```python
from build123d import *

# Parameters (mm, degrees)
F1_R     = 3.5625
F3_DEPTH = 12
F5_DEPTH = 3
F6_W     = 2.2875
F6_H     = 3.4472514316
F8_DEPTH = 2


with BuildPart() as f3:
    # F1 (on Top) → F3 (new body)
    with BuildSketch(Plane.XY):
        Circle(F1_R)
    extrude(amount=F3_DEPTH)

    # F2 (on Top) → F5 (join)
    with BuildSketch(Plane.XY):
        with BuildLine():
            ThreePointArc((-7.5208044782, -3), (-7.809575399, -2.1384648903), (-8, -1.25))
            ThreePointArc((-8, -1.25), (-9.25, 0), (-8, 1.25))
            ThreePointArc((-8, 1.25), (-7.809575399, 2.1384648903), (-7.5208044782, 3))
            Line((-7.5208044782, 3), (-9.25, 3))
            ThreePointArc((-9.25, 3), (-12.25, 0), (-9.25, -3))
            Line((-9.25, -3), (-7.5208044782, -3))
        make_face()
        with BuildLine():
            Line((-6, -1.25), (-8, -1.25))
            ThreePointArc((-8, -1.25), (-7.809575399, -2.1384648903), (-7.5208044782, -3))
            ThreePointArc((-7.5208044782, -3), (-5.7254912453, -5.7254912453), (-3, -7.5208044782))
            ThreePointArc((-3, -7.5208044782), (-2.1384648903, -7.809575399), (-1.25, -8))
            Line((-1.25, -8), (-1.25, -6))
            ThreePointArc((-1.25, -6), (0, -4.75), (1.25, -6))
            Line((1.25, -6), (1.25, -8))
            ThreePointArc((1.25, -8), (2.1384648903, -7.809575399), (3, -7.5208044782))
            ThreePointArc((3, -7.5208044782), (5.7254912453, -5.7254912453), (7.5208044782, -3))
            ThreePointArc((7.5208044782, -3), (7.809575399, -2.1384648903), (8, -1.25))
            Line((8, -1.25), (6, -1.25))
            ThreePointArc((6, -1.25), (4.75, 0), (6, 1.25))
            Line((6, 1.25), (8, 1.25))
            ThreePointArc((8, 1.25), (7.809575399, 2.1384648903), (7.5208044782, 3))
            ThreePointArc((7.5208044782, 3), (5.7254912453, 5.7254912453), (3, 7.5208044782))
            ThreePointArc((3, 7.5208044782), (2.1384648903, 7.809575399), (1.25, 8))
            Line((1.25, 8), (1.25, 6))
            ThreePointArc((1.25, 6), (0, 4.75), (-1.25, 6))
            Line((-1.25, 6), (-1.25, 8))
            ThreePointArc((-1.25, 8), (-2.1384648903, 7.809575399), (-3, 7.5208044782))
            ThreePointArc((-3, 7.5208044782), (-5.7254912453, 5.7254912453), (-7.5208044782, 3))
            ThreePointArc((-7.5208044782, 3), (-7.809575399, 2.1384648903), (-8, 1.25))
            Line((-8, 1.25), (-6, 1.25))
            ThreePointArc((-6, 1.25), (-4.75, 0), (-6, -1.25))
        make_face()
        with BuildLine():
            ThreePointArc((-1.25, -8), (-2.1384648903, -7.809575399), (-3, -7.5208044782))
            Line((-3, -7.5208044782), (-3, -9.25))
            ThreePointArc((-3, -9.25), (0, -12.25), (3, -9.25))
            Line((3, -9.25), (3, -7.5208044782))
            ThreePointArc((3, -7.5208044782), (2.1384648903, -7.809575399), (1.25, -8))
            ThreePointArc((1.25, -8), (0, -9.25), (-1.25, -8))
        make_face()
        with BuildLine():
            Line((-3, 9.25), (-3, 7.5208044782))
            ThreePointArc((-3, 7.5208044782), (-2.1384648903, 7.809575399), (-1.25, 8))
            ThreePointArc((-1.25, 8), (0, 9.25), (1.25, 8))
            ThreePointArc((1.25, 8), (2.1384648903, 7.809575399), (3, 7.5208044782))
            Line((3, 7.5208044782), (3, 9.25))
            ThreePointArc((3, 9.25), (0, 12.25), (-3, 9.25))
        make_face()
        with BuildLine():
            ThreePointArc((8, -1.25), (7.809575399, -2.1384648903), (7.5208044782, -3))
            Line((7.5208044782, -3), (9.25, -3))
            ThreePointArc((9.25, -3), (12.25, 0), (9.25, 3))
            Line((9.25, 3), (7.5208044782, 3))
            ThreePointArc((7.5208044782, 3), (7.809575399, 2.1384648903), (8, 1.25))
            ThreePointArc((8, 1.25), (9.25, 0), (8, -1.25))
        make_face()
    extrude(amount=-F5_DEPTH)

    # F6 (on Front) → F7 (revolve, cut)
    with BuildSketch(Plane.XZ):
        Polygon((0, -0.9375), (0, 0), (-1.35, 0), (-2.2875, -0.9375), align=None)
        Polygon((-1.35, 0), (0, 0), (0, 1.35), align=None)
        Polygon((-1.35, 17.6957350954), (-1.35, 0), (0, 1.35), (0, 17.6957350954), align=None)
        with Locations((-1.14375, -2.6611257158)):
            Rectangle(F6_W, F6_H)
    revolve(axis=Axis((0, 0, 8.8478675477), (0, 0, 1)), mode=Mode.SUBTRACT)

    # F4 (on face) → F8 (cut)
    with BuildSketch(Plane.XY.offset(12)):
        Polygon((1.5011106999, 2.6), (-1.5011106999, 2.6), (-3.0022213998, 0), (-1.5011106999, -2.6), (1.5011106999, -2.6), (3.0022213998, 0), align=None)
    extrude(amount=-F8_DEPTH, mode=Mode.SUBTRACT)


solid = f3.part
```
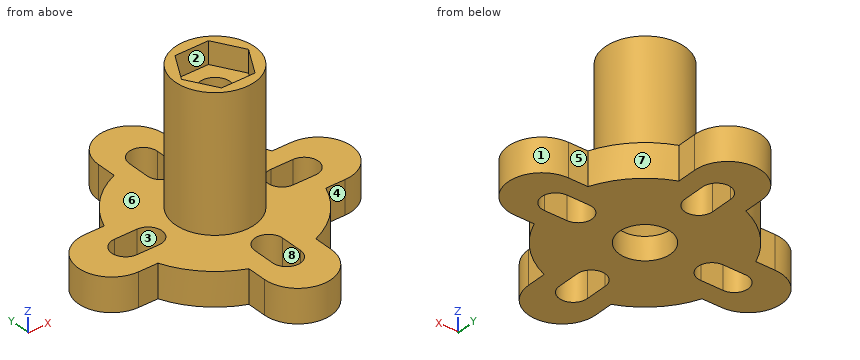
CAD build for the part. Positions are in the model's coordinates, mm. Face numbers are marked on the shaded views. A direction names the side the tool comes from. Round coordinates to 2 decimals unless told otherwise and drop trailing zeros. Order: outer loops, then holes, each group sorted by start corner. A loop starts at its lowest first (then second) coordinate and runs counter-clockwise, first axis right, second up.
Q1. Wall check: L1, parallel to Y at x = 0, z = -1.4; L2, parallel to Y at x = 0, z = 7.25. Give the ranges that are in metal, low to high.
Q2. Slice it at B-B (z = -1.75). State how many separate pieces and enclosed holes the cut face has, and give its area (3 significant figures).
Q3. Which spindle directions (+Z, -Z, +X, -X, +Y, -Y) get a long thin tool onto all of the face, cutting with end or side? Do the marked faces 1, 2, 3, 4 and 5. Say none if no direction does.
Q4. Two-plate mould, pull along Y, no slides. Class the marked faces 6, 7 and 8: pulls with the +Y half, pulls with the -Y half, needs draft (parallel to the pull), parting line crosses it, or undercut.
Q5. Slice it at C-C (y = 6.5). Write the cut outline in (x, z).
Q6. Drop flat-ended pins along their axis: pin 1 (0.6 mm diameter, centred on y = 7, z = -1.5, fed in from -X); pin 2 (2 mm diameter, centred on y = -7, z = -1.5, fed in from -X); pin 3 (1.6 mm diameter, centred on x = 0, y = 0, fed in from +Z); pin 4 (1.6 mm diameter, centred on y = 7, z = -1, fed in from +X). Give the stop position or say it passes through.
Q7. Slice it at A-A (x = 0). Write the cut outline in (y, z).
Results below:
1. L1: y = -12.25 to -9.25, -4.75 to -2.29, 2.29 to 4.75, 9.25 to 12.25
1. L2: y = -3.56 to -1.35, 1.35 to 3.56
2. separate pieces: 1
2. enclosed holes: 5
2. area: 239 mm2
3. face 1: +Z, -Z, +X
3. face 2: +Z
3. face 3: +Z, -Z
3. face 4: +Z, -Z, +X, -Y
3. face 5: +Z, -Z, +X, +Y
4. face 6: needs draft
4. face 7: pulls with the +Y half
4. face 8: undercut
5. outline: (-4.83, -3) - (-1.25, -3) - (-1.25, 0) - (-4.83, 0) - close; (1.25, -3) - (4.83, -3) - (4.83, 0) - (1.25, 0) - close
6. pin 1: stops at x = -4.55
6. pin 2: stops at x = -5.44
6. pin 3: passes through
6. pin 4: stops at x = 5.21
7. outline: (-12.25, -3) - (-9.25, -3) - (-9.25, 0) - (-12.25, 0) - close; (-4.75, -3) - (-2.29, -3) - (-2.29, -0.94) - (-1.35, 0) - (-1.35, 10) - (-2.6, 10) - (-2.6, 12) - (-3.56, 12) - (-3.56, 0) - (-4.75, 0) - close; (1.35, 0) - (2.29, -0.94) - (2.29, -3) - (4.75, -3) - (4.75, 0) - (3.56, 0) - (3.56, 12) - (2.6, 12) - (2.6, 10) - (1.35, 10) - close; (9.25, -3) - (12.25, -3) - (12.25, 0) - (9.25, 0) - close
